Work out the finished part from the listing and answer in its coordinate system (mm). Face numbers are marked on the shaded views. A direction names the side the tool comes from. Coordinates: 2 decimals unless noted, no trailing zeros. Loops run counter-clockwise (first coordinate to the right, second up) from the corner with the lowest first, then second, coordinate; pieces in that order, holes last. Notation, with made-up numbers: (84.5, 30) -> (115.5, 30) arc R18 cw to (115.5, 56) -> close; hole circle Ø1 at (31.5, -39.5). An arc over 180 degrees is marked (long way). One line per question, with ' | ' between items.
```python
from build123d import *

# Parameters (mm, degrees)
SKETCH_1_W          = 20
SKETCH_1_H          = 14
SKETCH_1_R          = 2.75
SKETCH_1_R_2        = 3.8
SKETCH_1_R_3        = 2.6
EXTRUDE_1_DEPTH     = 7
CUT_EXTRUDE_START   = -5
SKETCH_2_R          = 4.5
SKETCH_2_R_2        = 2.75
CUT_EXTRUDE_1_DEPTH = 5
SKETCH_8_R          = 1.25
CUT_EXTRUDE_3_DEPTH = 20.184368637
SKETCH_9_R          = 2.1
SKETCH_9_R_2        = 1.25
CUT_EXTRUDE_4_DEPTH = 6
EXTRUDE_START       = -4
EXTRUDE_2_DEPTH     = 4
SKETCH_11_W         = 1.5
SKETCH_11_H         = 4.7
EXTRUDE_3_DEPTH     = 1
CUT_EXTRUDE_5_DEPTH = 2
CUT_EXTRUDE_6_DEPTH = 1
FILLET_1_R          = 1
FILLET_2_R          = 0.5


with BuildPart() as part:
    # Эскиз1 → Бобышка-Вытянуть1 (new body)
    # profile 1 of 5: a face of its own
    with BuildSketch(Plane(origin=(0, 0, 0), x_dir=(1, 0, 0), z_dir=(0, 1, 0))):
        Rectangle(SKETCH_1_W, SKETCH_1_H)
        with Locations(Location((0, 0, 0), (0, 0, 270))):
            Circle(SKETCH_1_R, mode=Mode.SUBTRACT)
    # profile 2 of 5: a face of its own
    with BuildSketch(Plane(origin=(0, 0, 0), x_dir=(1, 0, 0), z_dir=(0, 1, 0))):
        with BuildLine():
            Line((-2.565353551, 13.803383877), (-10, 7))
            Line((-10, 7), (10, 7))
            Line((10, 7), (2.565353551, 13.803383877))
            ThreePointArc((2.565353551, 13.803383877), (3.477667573, 12.531609694), (3.8, 11))
            ThreePointArc((3.8, 11), (-1.531609694, 7.522332427), (-2.565353551, 13.803383877))
        make_face()
    # profile 3 of 5: a face of its own
    with BuildSketch(Plane(origin=(0, 0, 0), x_dir=(1, 0, 0), z_dir=(0, 1, 0))):
        with Locations((0, 11)):
            Circle(SKETCH_1_R_2)
        with Locations((0, 11)):
            Circle(SKETCH_1_R_3, mode=Mode.SUBTRACT)
    # profile 4 of 5: a face of its own
    with BuildSketch(Plane(origin=(0, 0, 0), x_dir=(1, 0, 0), z_dir=(0, 1, 0))):
        with BuildLine():
            ThreePointArc((1.112429773, 13.35), (0, 13.6), (-1.112429773, 13.35))
            Line((-1.112429773, 13.35), (1.112429773, 13.35))
        make_face()
    # profile 5 of 5: a face of its own
    with BuildSketch(Plane(origin=(0, 0, 0), x_dir=(1, 0, 0), z_dir=(0, 1, 0))):
        with BuildLine():
            Line((1.112429773, 8.65), (-1.112429773, 8.65))
            ThreePointArc((-1.112429773, 8.65), (0, 8.4), (1.112429773, 8.65))
        make_face()
    extrude(amount=EXTRUDE_1_DEPTH)

    # Эскиз2 → Вырез-Вытянуть1 (cut)
    with BuildSketch(Plane(origin=(0, 7, 0), x_dir=(1, 0, 0), z_dir=(0, 1, 0)).offset(CUT_EXTRUDE_START)):
        with Locations(Location((0, 0, 0), (0, 0, 270))):
            Circle(SKETCH_2_R)
        with Locations(Location((0, 0, 0), (0, 0, 270))):
            Circle(SKETCH_2_R_2, mode=Mode.SUBTRACT)
    extrude(amount=CUT_EXTRUDE_1_DEPTH, mode=Mode.SUBTRACT)

    # Эскиз8 → Вырез-Вытянуть3 (cut, through all)
    with BuildSketch(Plane(origin=(0, 7, 0), x_dir=(1, 0, 0), z_dir=(0, 1, 0))):
        with Locations(Location((7.2, 0, 0), (0, 0, 270))):
            Circle(SKETCH_8_R)
        with Locations(Location((-7.2, 0, 0), (0, 0, 90))):
            Circle(SKETCH_8_R)
    extrude(amount=-CUT_EXTRUDE_3_DEPTH, mode=Mode.SUBTRACT)

    # Эскиз9 → Вырез-Вытянуть4 (cut)
    # profile 1 of 2: a face of its own
    with BuildSketch(Plane(origin=(0, 7, 0), x_dir=(1, 0, 0), z_dir=(0, 1, 0))):
        with Locations(Location((-7.2, 0, 0), (0, 0, 270))):
            Circle(SKETCH_9_R)
        with Locations(Location((-7.2, 0, 0), (0, 0, 270))):
            Circle(SKETCH_9_R_2, mode=Mode.SUBTRACT)
    # profile 2 of 2: a face of its own
    with BuildSketch(Plane(origin=(0, 7, 0), x_dir=(1, 0, 0), z_dir=(0, 1, 0))):
        with Locations(Location((7.2, 0, 0), (0, 0, 270))):
            Circle(SKETCH_9_R)
        with Locations(Location((7.2, 0, 0), (0, 0, 270))):
            Circle(SKETCH_9_R_2, mode=Mode.SUBTRACT)
    extrude(amount=-CUT_EXTRUDE_4_DEPTH, mode=Mode.SUBTRACT)

    # Эскиз10 → Бобышка-Вытянуть2 (add)
    with BuildSketch(Plane(origin=(0, 7, 0), x_dir=(1, 0, 0), z_dir=(0, 1, 0)).offset(EXTRUDE_START)):
        with BuildLine():
            ThreePointArc((1.112429773, 13.35), (2.6, 11), (1.112429773, 8.65))
            Line((1.112429773, 8.65), (-1.112429773, 8.65))
            ThreePointArc((-1.112429773, 8.65), (-2.6, 11), (-1.112429773, 13.35))
            Line((-1.112429773, 13.35), (1.112429773, 13.35))
        make_face()
    extrude(amount=EXTRUDE_2_DEPTH)

    # Эскиз11 → Бобышка-Вытянуть3 (add)
    with BuildSketch(Plane.XZ.offset(-3)):
        with Locations((0, -11)):
            Rectangle(SKETCH_11_W, SKETCH_11_H)
    extrude(amount=EXTRUDE_3_DEPTH)

    # Эскиз12 → Вырез-Вытянуть5 (cut)
    with BuildSketch(Plane.XZ):
        Polygon((-2, -5.5), (-2, -8.65), (-1.112429773, -8.65), (1.112429773, -8.65), (2, -8.65), (2, -5.5), align=None)
        with BuildLine():
            Line((-1.112429773, -8.65), (-2, -8.65))
            Line((-2, -8.65), (-2, -9.338675227))
            ThreePointArc((-2, -9.338675227), (-1.593854813, -8.945826971), (-1.112429773, -8.65))
        make_face()
        with BuildLine():
            Line((2, -8.65), (1.112429773, -8.65))
            ThreePointArc((1.112429773, -8.65), (1.593854813, -8.945826971), (2, -9.338675227))
            Line((2, -9.338675227), (2, -8.65))
        make_face()
    extrude(amount=-CUT_EXTRUDE_5_DEPTH, mode=Mode.SUBTRACT)

    # Эскиз13 → Вырез-Вытянуть6 (cut)
    with BuildSketch(Plane.XZ.offset(-2)):
        with BuildLine():
            Line((2, -5.5), (0.75, -5.5))
            Line((0.75, -5.5), (0.75, -8.65))
            Line((0.75, -8.65), (1.112429773, -8.65))
            ThreePointArc((1.112429773, -8.65), (1.593854813, -8.945826971), (2, -9.338675227))
            Line((2, -9.338675227), (2, -5.5))
        make_face()
        with BuildLine():
            Line((-1.112429773, -8.65), (-0.75, -8.65))
            Line((-0.75, -8.65), (-0.75, -5.5))
            Line((-0.75, -5.5), (-2, -5.5))
            Line((-2, -5.5), (-2, -9.338675227))
            ThreePointArc((-2, -9.338675227), (-1.593854813, -8.945826971), (-1.112429773, -8.65))
        make_face()
    extrude(amount=-CUT_EXTRUDE_6_DEPTH, mode=Mode.SUBTRACT)

    # Скругление1
    fillet_1_edges = [part.edges().sort_by_distance(p)[0] for p in [
        (-10, 3.5, 7),
        (-10, 3.5, -7),
        (10, 3.5, -7),
        (10, 3.5, 7),
    ]]
    fillet(fillet_1_edges, radius=FILLET_1_R)

    # Скругление2
    # the kernel refuses this fillet: 0.5 mm, written as the material it takes off along each edge
    with BuildSketch(Plane(origin=(-10, 7, -6.559587091), x_dir=(1, 0, 0), z_dir=(0, 0, 1)), Plane(origin=(10, 7, 6), x_dir=(-1, 0, 0), z_dir=(0, 0, -1))) as fillet_2_piece_1:
        with BuildLine():
            CenterArc((FILLET_2_R, -FILLET_2_R), FILLET_2_R, 90, 90)
            Line((0, -FILLET_2_R), (0, 0))
            Line((0, 0), (FILLET_2_R, 0))
        make_face()
    extrude(amount=12.559587091, mode=Mode.SUBTRACT)
    with BuildSketch(Plane(origin=(-2.565353551, 7, -13.803383877), x_dir=(0.6750930396508724, 0, 0.7377325991271809), z_dir=(-0.7377325991271809, 0, 0.6750930396508723)), Plane(origin=(9.67509304, 7, -7.29731969), x_dir=(-0.6750930396508725, 0, 0.7377325991271807), z_dir=(-0.7377325991271807, 0, -0.6750930396508726))) as fillet_2_piece_2:
        with BuildLine():
            CenterArc((FILLET_2_R, -FILLET_2_R), FILLET_2_R, 90, 90)
            Line((0, -FILLET_2_R), (0, 0))
            Line((0, 0), (FILLET_2_R, 0))
        make_face()
    extrude(amount=9.63728524, mode=Mode.SUBTRACT)
    with BuildSketch(Plane(origin=(-9, 7, 7), x_dir=(0, -1, 0), z_dir=(1, 0, 0))) as fillet_2_piece_3:
        with BuildLine():
            CenterArc((FILLET_2_R, FILLET_2_R), FILLET_2_R, 180, 90)
            Line((0, FILLET_2_R), (0, 0))
            Line((0, 0), (FILLET_2_R, 0))
        make_face()
    extrude(amount=18, mode=Mode.SUBTRACT)
    with BuildSketch(Plane(origin=(9, 7, -6.559587091), x_dir=(0.6750930396508728, 0, -0.7377325991271806), z_dir=(-0.7377325991271806, 0, -0.6750930396508728))) as fillet_2_piece_4:
        with BuildLine():
            CenterArc((1 - FILLET_2_R, FILLET_2_R), FILLET_2_R, 270, 90)
            Line((1, FILLET_2_R), (1, 0))
            Line((1, 0), (1 - FILLET_2_R, 0))
        make_face()
    revolve(axis=Axis((9, 7, -6.559587091), (0, -1, 0)), revolution_arc=47.538624316, mode=Mode.SUBTRACT)
    with BuildSketch(Plane(origin=(9, 7, 6), x_dir=(0, 0, 1), z_dir=(-1, 0, 0))) as fillet_2_piece_5:
        with BuildLine():
            CenterArc((1 - FILLET_2_R, -FILLET_2_R), FILLET_2_R, 0, 90)
            Line((1 - FILLET_2_R, 0), (1, 0))
            Line((1, 0), (1, -FILLET_2_R))
        make_face()
    revolve(axis=Axis((9, 7, 6), (0, 1, 0)), revolution_arc=90, mode=Mode.SUBTRACT)
    with BuildSketch(Plane(origin=(-9, 7, 6), x_dir=(0, 0, 1), z_dir=(1, 0, 0))) as fillet_2_piece_6:
        with BuildLine():
            CenterArc((1 - FILLET_2_R, FILLET_2_R), FILLET_2_R, 270, 90)
            Line((1 - FILLET_2_R, 0), (1, 0))
            Line((1, 0), (1, FILLET_2_R))
        make_face()
    revolve(axis=Axis((-9, 7, 6), (0, -1, 0)), revolution_arc=90, mode=Mode.SUBTRACT)
    with BuildSketch(Plane(origin=(-9, 7, -6.559587091), x_dir=(-0.6750930396508718, 0, -0.7377325991271815), z_dir=(0.7377325991271815, 0, -0.6750930396508718))) as fillet_2_piece_7:
        with BuildLine():
            CenterArc((1 - FILLET_2_R, -FILLET_2_R), FILLET_2_R, 0, 90)
            Line((1, -FILLET_2_R), (1, 0))
            Line((1, 0), (1 - FILLET_2_R, 0))
        make_face()
    revolve(axis=Axis((-9, 7, -6.559587091), (0, 1, 0)), revolution_arc=47.538624316, mode=Mode.SUBTRACT)
    with BuildSketch(Plane(origin=(0, 7, -11), x_dir=(0.6750930396508724, 0, -0.7377325991271808), z_dir=(0.7377325991271808, 0, 0.6750930396508724))) as fillet_2_piece_8:
        with BuildLine():
            CenterArc((3.8 - FILLET_2_R, -FILLET_2_R), FILLET_2_R, 0, 90)
            Line((3.8, -FILLET_2_R), (3.8, 0))
            Line((3.8, 0), (3.8 - FILLET_2_R, 0))
        make_face()
    revolve(axis=Axis((0, 7, -11), (0, 1, 0)), revolution_arc=84.922751368, mode=Mode.SUBTRACT)
    with BuildSketch(Plane(origin=(0, 7, 0), x_dir=(0, 0, 1), z_dir=(-1, 0, 0))) as fillet_2_piece_9:
        with BuildLine():
            CenterArc((4.5 + FILLET_2_R, -FILLET_2_R), FILLET_2_R, 90, 90)
            Line((4.5, -FILLET_2_R), (4.5, 0))
            Line((4.5, 0), (4.5 + FILLET_2_R, 0))
        make_face()
    revolve(axis=Axis((0, 7, 0), (0, 1, 0)), mode=Mode.SUBTRACT)
    with BuildSketch(Plane(origin=(-7.2, 7, 0), x_dir=(0, 0, 1), z_dir=(-1, 0, 0))) as fillet_2_piece_10:
        with BuildLine():
            CenterArc((2.1 + FILLET_2_R, -FILLET_2_R), FILLET_2_R, 90, 90)
            Line((2.1, -FILLET_2_R), (2.1, 0))
            Line((2.1, 0), (2.1 + FILLET_2_R, 0))
        make_face()
    revolve(axis=Axis((-7.2, 7, 0), (0, 1, 0)), mode=Mode.SUBTRACT)
    with BuildSketch(Plane(origin=(7.2, 7, 0), x_dir=(0, 0, 1), z_dir=(-1, 0, 0))) as fillet_2_piece_11:
        with BuildLine():
            CenterArc((2.1 + FILLET_2_R, -FILLET_2_R), FILLET_2_R, 90, 90)
            Line((2.1, -FILLET_2_R), (2.1, 0))
            Line((2.1, 0), (2.1 + FILLET_2_R, 0))
        make_face()
    revolve(axis=Axis((7.2, 7, 0), (0, 1, 0)), mode=Mode.SUBTRACT)


solid = part.part
```
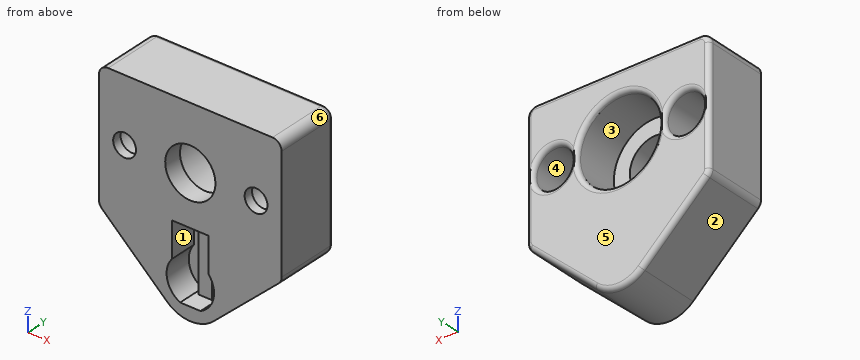
1) Find section B-B (y = 2.5). Write down the section's boundary in (x, z).
Check values:
outline: (-10, -6.56) arc R1 ccw to (-9.68, -7.3) -> (-2.57, -13.8) arc R3.8 ccw to (2.57, -13.8) -> (9.68, -7.3) arc R1 ccw to (10, -6.56) -> (10, 6) arc R1 ccw to (9, 7) -> (-9, 7) arc R1 ccw to (-10, 6) -> close; hole circle Ø4.2 at (-7.2, 0); hole circle Ø9 at (0, 0); hole (-2, -9.34) arc R2.6 ccw to (-1.11, -13.35) -> (-0.75, -13.35) -> (-0.75, -5.5) -> (-2, -5.5) -> close; hole (0.75, -13.35) -> (1.11, -13.35) arc R2.6 ccw to (2, -9.34) -> (2, -5.5) -> (0.75, -5.5) -> close; hole circle Ø4.2 at (7.2, 0)
2) Find section A-A (x = 0). Write down the section's boundary in (y, z).
Check values:
outline: (0, -14.8) -> (6.5, -14.8) arc R0.5 ccw to (7, -14.3) -> (7, -5) arc R0.5 ccw to (6.5, -4.5) -> (2, -4.5) -> (2, -2.75) -> (0, -2.75) -> (0, -5.5) -> (2, -5.5) -> (2, -13.35) -> (0, -13.35) -> close; (0, 2.75) -> (2, 2.75) -> (2, 4.5) -> (6.5, 4.5) arc R0.5 ccw to (7, 5) -> (7, 6.5) arc R0.5 ccw to (6.5, 7) -> (0, 7) -> close
3) Find section D-D (z = 0). State how many separate pieces and enclosed holes the cut face has, plus the area to 3 significant figures.
Check values:
separate pieces: 4 | enclosed holes: 0 | area: 28.2 mm^2
4) The mould has two halves that part along Z. Classify the marked faces 4, 5 and 6: released by +Z, released by -Z, zero draft, split by the parting line, or undercut.
Check values:
face 4: undercut | face 5: zero draft | face 6: released by +Z
5) For the marked faces 1, 2 and 3, determine the directions among +Z, -Z, +X, -X, +Y, -Y from which every point of the face is accessible in a straight line to the end or side of a thin tool.
Check values:
face 1: -Y | face 2: -Z, -X, +Y, -Y | face 3: +Y
6) Flat-ended cylindrical pins translate along their axes: pin 1 (3.5 mm diameter, centred on y = 1, z = -8.5, fed in from -X); pin 2 (3 mm diameter, centred on x = -5, y = 1.5, fed in from -Z); pin 3 (2 mm diameter, centred on y = 5, z = -12, fed in from -X). Find the tip coordinate at first contact, or state that the pin passes through.
Check values:
pin 1: stops at x = -9.98 | pin 2: stops at z = -12.95 | pin 3: stops at x = -5.63
7) Find the intervals of material crossed by line 1 along X through (y, z) = (0.45, 0); line 2 along X through (y, z) = (5.05, 0); line 3 along Z through (x, y) = (-7.2, 0.4), in increasing order.
Check values:
line 1: x = -10 to -8.45, -5.95 to -2.75, 2.75 to 5.95, 8.45 to 10 | line 2: x = -10 to -9.3, -5.1 to -4.5, 4.5 to 5.1, 9.3 to 10 | line 3: z = -9.56 to -1.25, 1.25 to 7
8) Find section C-C (y = 4.75). Write down the section's boundary in (x, z), plus the area to 3 significant figures.
Check values:
outline: (-10, -6.56) arc R1 ccw to (-9.68, -7.3) -> (-2.57, -13.8) arc R3.8 ccw to (2.57, -13.8) -> (9.68, -7.3) arc R1 ccw to (10, -6.56) -> (10, 6) arc R1 ccw to (9, 7) -> (-9, 7) arc R1 ccw to (-10, 6) -> close; hole circle Ø4.2 at (-7.2, 0); hole circle Ø9 at (0, 0); hole circle Ø4.2 at (7.2, 0) | area: 277 mm^2
